Geometry: final body of the model. Coordinates: model frame, mm. Give positions to 0.01 mm unless a question says otherwise; leave off trailing zeros. Write each loop counter-clockwise with the first axis right and the second up, starting at its lowest first coordinate (ties: lowest second). Pieces come first, ordered by that corner, then holes. Notation, with made-up numbers: M 21,53 L 63,53 A22 ccw 63,61 Z; hole C 86.5,37 d10. An arc over 180 degrees is marked long. One line per question, with ' | ' between items.
from build123d import *

# Parameters (mm, degrees)
CYLINDER026_R     = 10.5
CYLINDER026_DEPTH = 13
CYLINDER025_R     = 12
CYLINDER025_DEPTH = 7


with BuildPart() as cylinder026:
    # Cylinder026 → Cylinder026 (new body)
    with BuildSketch(Plane.XY.offset(-6)):
        Circle(CYLINDER026_R)
    extrude(amount=CYLINDER026_DEPTH)


with BuildPart() as cut094:
    # Cylinder025 → Cylinder025 (new body)
    with BuildSketch(Plane.XY.offset(-6)):
        Circle(CYLINDER025_R)
    extrude(amount=CYLINDER025_DEPTH)

    # Cut094: cut Cylinder026
    add(cylinder026.part, mode=Mode.SUBTRACT)


solid = cut094.part
(1) Draft query along Y for faces 1 (the face through (10, 3.2, -2.5)), 2 (the face through (-11.99, 0.53, -2.55)), 3 (the face through (0, -11, 1)). Return one class per face: released by +Y, released by -Y, zero draft, split by the parting line, or undercut.
Working result:
face 1: undercut | face 2: split by the parting line | face 3: zero draft
(2) Cut plane B-B, the plane x = 6. Return loops of the section in (y, z).
Working result:
outline: M -10.39,-6 L -8.62,-6 L -8.62,1 L -10.39,1 Z; M 8.62,-6 L 10.39,-6 L 10.39,1 L 8.62,1 Z
(3) Cut plane C-C, the plane z = -2.25. Return loops of the section in (x, y), then the cut area to 3 significant figures.
Working result:
outline: C 0,0 d24; hole C 0,0 d21 | area: 106 mm^2
(4) Cut plane A-A, the plane y = 0. Return loops of the section in (x, z), then the cut area to 3 significant figures.
Working result:
outline: M -12,-6 L -10.5,-6 L -10.5,1 L -12,1 Z; M 10.5,-6 L 12,-6 L 12,1 L 10.5,1 Z | area: 21.0 mm^2
(5) Material intervals for L1, parallel to Y at x = 0, z = -3; L2, parallel to X at y = 7.5, z = -3.5; L3, parallel to Y at x = -1.5, z = -0.5, sorted ascending. Write a range as [from, to].
Working result:
L1: y = [-12, -10.5], [10.5, 12] | L2: x = [-9.37, -7.35], [7.35, 9.37] | L3: y = [-11.91, -10.39], [10.39, 11.91]
(6) First-contact query: P1, Ø3, axis at x = -7, z = -5, coming from the -Y side; P2, Ø1.5, axis at y = -1.5, z = -5, coming from the +X side; P3, Ø6, axis at x = -2.5, y = -8.5, coming from the -Z side; P4, Ø1.5, axis at x = -2.5, z = -1.5, coming from the +Y side. Flat tips, straight axial feed; report the tip coordinate or a pass-through.
Working result:
P1: stops at y = -10.67 | P2: stops at x = 11.98 | P3: stops at z = -6 | P4: stops at y = 11.87
